Part model, mm, in its own coordinate system. A direction names the side the tool comes from. Give positions to 0.01 mm unless a question says otherwise; leave off trailing zeros. Loops run counter-clockwise (first coordinate to the right, second up) from the corner with the lowest first, then second, coordinate; pieces in that order, holes last. Notation, with made-up numbers: (-11, 15) -> (20, 15) arc R26 ccw to (20, 37) -> close; hole circle Ø3 at (-25, -31.75). An arc over 180 degrees is marked (long way). Write item = value, one per line.
from build123d import *

# Parameters (mm, degrees)
F0_W     = 12.7
F0_H     = 6.35
F0_R     = 20
F1_DEPTH = 6.35
F3_DEPTH = 25.4
F4_R     = 1.27
F5_DEPTH = 25.4


with BuildPart() as f1:
    # F0 (on Top) → F1 (new body)
    with BuildSketch(Plane.XY):
        Polygon((-48.26, 101.6), (-63.5, 101.6), (-63.5, 50.8), (-63.5, -50.8), (-63.5, -101.6), (-48.26, -101.6), (-35.56, -101.6), (35.56, -101.6), (48.26, -101.6), (63.5, -101.6), (63.5, -50.8), (63.5, 50.8), (63.5, 101.6), (48.26, 101.6), (35.56, 101.6), (-35.56, 101.6), align=None)
        with Locations((-41.91, 104.775)):
            Rectangle(F0_W, F0_H)
        with BuildLine():
            Line((-63.5, -50.8), (-63.5, 50.8))
            Line((-63.5, 50.8), (-115.958545, 31.706651))
            ThreePointArc((-115.958545, 31.706651), (-92.443608, 23.02956), (-82.55, 0))
            ThreePointArc((-82.55, 0), (-92.443608, -23.02956), (-115.958545, -31.706651))
            Line((-115.958545, -31.706651), (-63.5, -50.8))
        make_face()
        with BuildLine():
            ThreePointArc((-82.55, 0), (-92.443608, 23.02956), (-115.958545, 31.706651))
            ThreePointArc((-115.958545, 31.706651), (-146.05, 0), (-115.958545, -31.706651))
            ThreePointArc((-115.958545, -31.706651), (-92.443608, -23.02956), (-82.55, 0))
        make_face()
        with Locations((-114.3, 0)):
            Circle(F0_R, mode=Mode.SUBTRACT)
        with Locations((41.91, 104.775)):
            Rectangle(F0_W, F0_H)
        with Locations((-41.91, -104.775)):
            Rectangle(F0_W, F0_H)
        with BuildLine():
            Line((115.958545, 31.706651), (63.5, 50.8))
            Line((63.5, 50.8), (63.5, -50.8))
            Line((63.5, -50.8), (115.958545, -31.706651))
            ThreePointArc((115.958545, -31.706651), (82.55, 0), (115.958545, 31.706651))
        make_face()
        with Locations((41.91, -104.775)):
            Rectangle(F0_W, F0_H)
        with BuildLine():
            ThreePointArc((146.05, 0), (137.32956, 21.856392), (115.958545, 31.706651))
            ThreePointArc((115.958545, 31.706651), (82.55, 0), (115.958545, -31.706651))
            ThreePointArc((115.958545, -31.706651), (137.32956, -21.856392), (146.05, 0))
        make_face()
        with Locations((114.3, 0)):
            Circle(F0_R, mode=Mode.SUBTRACT)
    extrude(amount=F1_DEPTH)

    # F2 (on face) → F3 (cut)
    with BuildSketch(Plane.XY.offset(6.35)):
        with BuildLine():
            ThreePointArc((-28.743891, 79.535165), (-26.683078, 78.157131), (-24.251671, 77.6732))
            Line((-24.251671, 77.6732), (-10.16, 77.6732))
            Line((-10.16, 77.6732), (-10.16, 88.9))
            Line((-10.16, 88.9), (-38.1, 88.9))
            Line((-38.1, 88.9), (-28.743891, 79.535165))
        make_face()
        with BuildLine():
            Line((-10.16, -75.875254), (-23.971951, -75.875254))
            ThreePointArc((-23.971951, -75.875254), (-26.61868, -76.453137), (-28.783676, -78.081608))
            Line((-28.783676, -78.081608), (-38.1, -88.9))
            Line((-38.1, -88.9), (-10.16, -88.9))
            Line((-10.16, -88.9), (-10.16, -75.875254))
        make_face()
        with BuildLine():
            Line((23.98423, -75.875254), (10.16, -75.875254))
            Line((10.16, -75.875254), (10.16, -88.9))
            Line((10.16, -88.9), (38.1, -88.9))
            Line((38.1, -88.9), (28.798656, -78.084747))
            ThreePointArc((28.798656, -78.084747), (26.632841, -76.454001), (23.98423, -75.875254))
        make_face()
        with BuildLine():
            Line((41.353395, -66.799067), (50.8, -76.2))
            Line((50.8, -76.2), (50.8, -16.477037))
            ThreePointArc((50.8, -16.477037), (49.684077, -13.78296), (46.99, -12.667037))
            Line((46.99, -12.667037), (43.399565, -12.667037))
            ThreePointArc((43.399565, -12.667037), (40.708633, -13.779818), (39.589575, -16.468145))
            Line((39.589575, -16.468145), (39.482647, -62.283251))
            ThreePointArc((39.482647, -62.283251), (39.966103, -64.728373), (41.353395, -66.799067))
        make_face()
        with BuildLine():
            Line((-50.8, -14.712054), (-50.8, -76.2))
            Line((-50.8, -76.2), (-41.121936, -64.961544))
            ThreePointArc((-41.121936, -64.961544), (-39.980638, -63.027881), (-39.583661, -60.817898))
            Line((-39.583661, -60.817898), (-39.583661, -14.712054))
            ThreePointArc((-39.583661, -14.712054), (-40.699584, -12.017977), (-43.393661, -10.902054))
            Line((-43.393661, -10.902054), (-46.99, -10.902054))
            ThreePointArc((-46.99, -10.902054), (-49.684077, -12.017977), (-50.8, -14.712054))
        make_face()
        with BuildLine():
            Line((50.8, 16.51), (50.8, 76.2))
            Line((50.8, 76.2), (41.453267, 66.832201))
            ThreePointArc((41.453267, 66.832201), (40.080445, 64.773868), (39.598446, 62.34713))
            Line((39.598446, 62.34713), (39.598446, 16.51))
            ThreePointArc((39.598446, 16.51), (40.714369, 13.815923), (43.408446, 12.7))
            Line((43.408446, 12.7), (46.99, 12.7))
            ThreePointArc((46.99, 12.7), (49.684077, 13.815923), (50.8, 16.51))
        make_face()
        with BuildLine():
            Line((10.16, 88.9), (10.16, 77.6732))
            Line((10.16, 77.6732), (24.251671, 77.6732))
            ThreePointArc((24.251671, 77.6732), (26.683078, 78.157131), (28.743891, 79.535165))
            Line((28.743891, 79.535165), (38.1, 88.9))
            Line((38.1, 88.9), (10.16, 88.9))
        make_face()
        with BuildLine():
            Line((-41.44144, 66.832712), (-50.8, 76.2))
            Line((-50.8, 76.2), (-50.8, 13.881477))
            ThreePointArc((-50.8, 13.881477), (-49.684077, 11.187401), (-46.99, 10.071477))
            Line((-46.99, 10.071477), (-43.393661, 10.071477))
            ThreePointArc((-43.393661, 10.071477), (-40.699584, 11.187401), (-39.583661, 13.881477))
            Line((-39.583661, 13.881477), (-39.583661, 62.344677))
            ThreePointArc((-39.583661, 62.344677), (-40.066459, 64.77335), (-41.44144, 66.832712))
        make_face()
    extrude(amount=-F3_DEPTH, mode=Mode.SUBTRACT)

    # F4 (on face) → F5 (cut)
    with BuildSketch(Plane.XY.offset(6.35)):
        with BuildLine():
            ThreePointArc((30.687634, -52.062728), (31.957634, -53.332728), (33.227634, -52.062728))
            ThreePointArc((33.227634, -52.062728), (31.957634, -50.792728), (30.687634, -52.062728))
        make_face()
        with Locations((-30.42054, -52.062728)):
            Circle(F4_R)
        with BuildLine():
            ThreePointArc((-30.849525, -0.579722), (-32.119525, 0.690278), (-33.389525, -0.579722))
            Line((-33.389525, -0.579722), (-30.849525, -0.579722))
        make_face()
        with BuildLine():
            ThreePointArc((35.97056, -0.579722), (34.70056, 0.690278), (33.43056, -0.579722))
            Line((33.43056, -0.579722), (35.97056, -0.579722))
        make_face()
        with BuildLine():
            Line((35.97056, -0.579722), (33.43056, -0.579722))
            ThreePointArc((33.43056, -0.579722), (34.70056, -1.849722), (35.97056, -0.579722))
        make_face()
        with BuildLine():
            Line((-30.849525, -0.579722), (-33.389525, -0.579722))
            ThreePointArc((-33.389525, -0.579722), (-32.119525, -1.849722), (-30.849525, -0.579722))
        make_face()
    extrude(amount=-F5_DEPTH, mode=Mode.SUBTRACT)


solid = f1.part
1) Drop flat-ended pins along their axis: P1, Ø1.9, axis at y = 104, z = 4, coming from the -X side; P2, Ø1.9, axis at x = -52.5, z = 3, coming from the -Y side; P3, Ø8, axis at x = 43, y = 43, coming from the +Z side; P4, Ø1.5, axis at y = -75.5, z = 5.5, coming from the +X side. Give the stop position or say it passes through.
Resolved:
P1 = -48.26
P2 = -101.6
P3 = 6.35
P4 = 63.5
2) Which spindle directions (+Z, -Z, +X, -X, +Y, -Y) get a long thin tool onto all of the face, cutting with end or side? Do faces 4 (the face through (-35.56, 105, 3)), 5 (the face through (39.598, 40, 3)), 6 (the face through (-2, 2, 6.35)), 7 (the face through (56, 101.6, 3)), 8 (the face through (-48.26, -105, 3)). Say none if no direction does.
Resolved:
face_4 = +Z, -Z, +Y
face_5 = +Z, -Z
face_6 = +Z, +X, -X, +Y, -Y
face_7 = +Z, -Z, +X, +Y
face_8 = +Z, -Z, -X, -Y
3) Slice it at B-B, the plane y = -72.5. List the corners of the cut face in (x, z), and give its area (3 significant figures).
Resolved:
outline = (-63.5, 0) -> (-50.8, 0) -> (-50.8, 6.35) -> (-63.5, 6.35) -> close; (-47.61, 0) -> (47.08, 0) -> (47.08, 6.35) -> (-47.61, 6.35) -> close; (50.8, 0) -> (63.5, 0) -> (63.5, 6.35) -> (50.8, 6.35) -> close
area = 763 mm²
4) Slice it at D-D, the plane z = 1. Count the separate pieces of the cut face and the enclosed holes in it, and give its area (3 significant figures).
Resolved:
separate_pieces = 1
enclosed_holes = 14
area = 31,500 mm²
5) Slice it at A-A, the plane y = 56. List the corners of the cut face in (x, z).
Resolved:
outline = (-63.5, 0) -> (-50.8, 0) -> (-50.8, 6.35) -> (-63.5, 6.35) -> close; (-39.58, 0) -> (39.6, 0) -> (39.6, 6.35) -> (-39.58, 6.35) -> close; (50.8, 0) -> (63.5, 0) -> (63.5, 6.35) -> (50.8, 6.35) -> close
6) Pull direction Y, two halves, no side cores. Call faces 1 (the face through (90.1, 41.12, 3.13)), 2 (the face through (35.56, -105, 3)), 3 (the face through (-50.8, -45, 3)): pulls with the +Y half, pulls with the -Y half, needs draft (parallel to the pull), parting line crosses it, or undercut.
Resolved:
face_1 = pulls with the +Y half
face_2 = needs draft
face_3 = undercut
7) Drill centre lines: line 1 along X through (y, z) = (-58, 4); line 2 along X through (y, z) = (51.5, 5.75); line 3 along Y through (x, z) = (18, 1.5). Where is each one in solid material? Low to high. Write a range as [from, to].
Resolved:
line_1 = [-63.5, -50.8], [-39.58, 39.49], [50.8, 63.5]
line_2 = [-63.5, -50.8], [-39.58, 39.6], [50.8, 63.5]
line_3 = [-101.6, -88.9], [-75.88, 77.67], [88.9, 101.6]
8) Slice it at C-C, the plane x = 56.5. List the corners of the cut face in (y, z), and give its area (3 significant figures).
Resolved:
outline = (-101.6, 0) -> (101.6, 0) -> (101.6, 6.35) -> (-101.6, 6.35) -> close
area = 1,290 mm²
